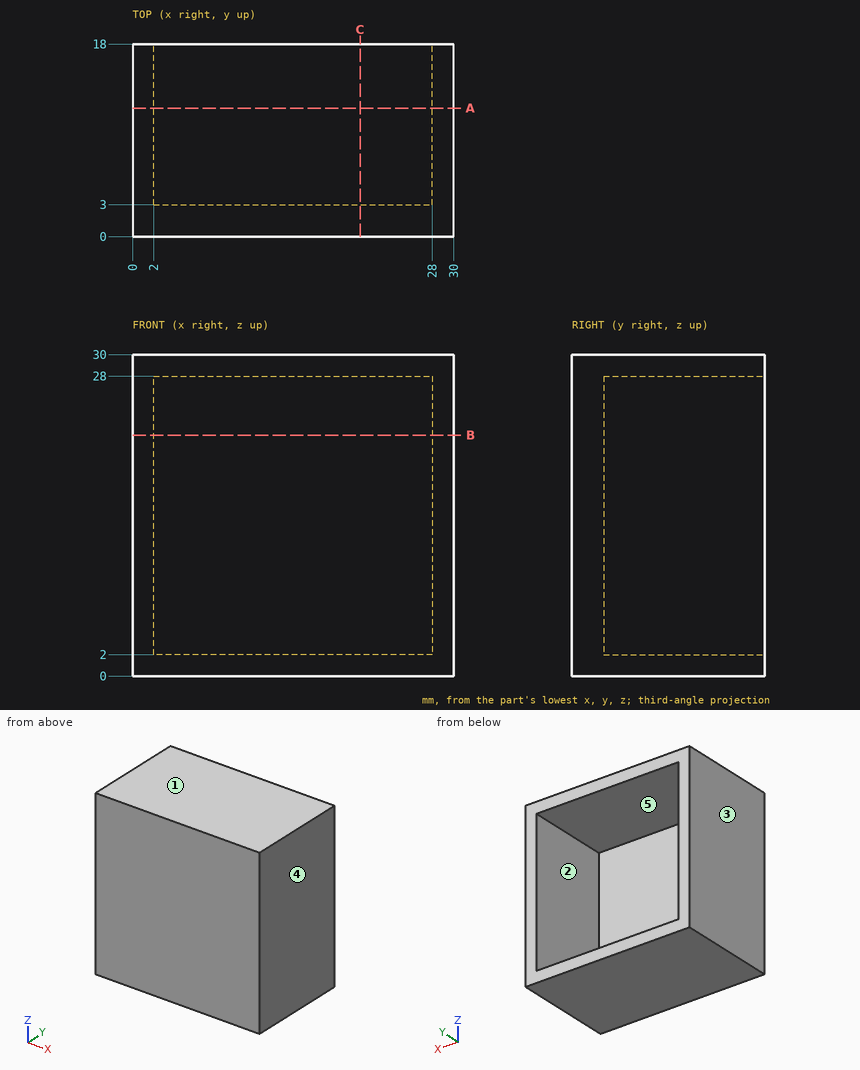
The drawing under review shows one solid part. Ordinate dimensions are in mm from its lowest x, y, z. A direction names the side the tool comes from. Coordinates: 2 decimals unless noted, no trailing zeros. Order: outer loops, then holes, each group sorted by start corner. A loop starts at its lowest first (then second) coordinate and runs counter-clockwise, first axis right, second up. Notation, with made-up numbers: (34, 81) - (44, 81) arc R34 cw to (44, 115) - close; hole circle Ø9 at (74, 60). An arc over 180 degrees is marked (long way). Put each result on its own line as item: value.
1) The part is to be moulded in two halves that separate along Z. For the marked faces 1, 2 and 3, say which applies: released by +Z, released by -Z, zero draft, split by the parting line, or undercut.
Response values:
face 1: released by +Z
face 2: undercut
face 3: zero draft
2) Take a section at A-A, the plane y = 12. Give the boundary of the cut face in (x, z).
Response values:
outline: (0, 0) - (30, 0) - (30, 30) - (0, 30) - close; hole (2, 2) - (28, 2) - (28, 28) - (2, 28) - close
3) Take a section at B-B, the plane z = 22.5. Give the boundary of the cut face in (x, y).
Response values:
outline: (0, 0) - (30, 0) - (30, 18) - (28, 18) - (28, 3) - (2, 3) - (2, 18) - (0, 18) - close
4) Take a section at C-C, the plane x = 21.25. Give the boundary of the cut face in (y, z).
Response values:
outline: (0, 0) - (18, 0) - (18, 2) - (3, 2) - (3, 28) - (18, 28) - (18, 30) - (0, 30) - close
5) Tool access review of the marked faces 4 and 5: name each direction out of +Z, -Z, +X, -X, +Y, -Y from which nothing blocks a thin tool from reaching the whole face with its end or side.
Response values:
face 4: +Z, -Z, +X, +Y, -Y
face 5: +Y
6) Wall thickness on L1, parallel to X at y = 13, z = 19.75; L2, parallel to Y at x = 18.25, z = 11: over which ranges is each line inside the solid? List them lowest first. Write a range as from..to.
Response values:
L1: x = 0..2, 28..30
L2: y = 0..3
7) Insertion check: P1, Ø1.5, axis at x = 9.5, y = 3.5, coming from the -Z side; P2, Ø13, axis at x = 19.5, z = 18, coming from the +Y side. Each pin has a flat end and moves straight along its axis. Give the tip position at first contact, or say it passes through.
Response values:
P1: stops at z = 0
P2: stops at y = 3
